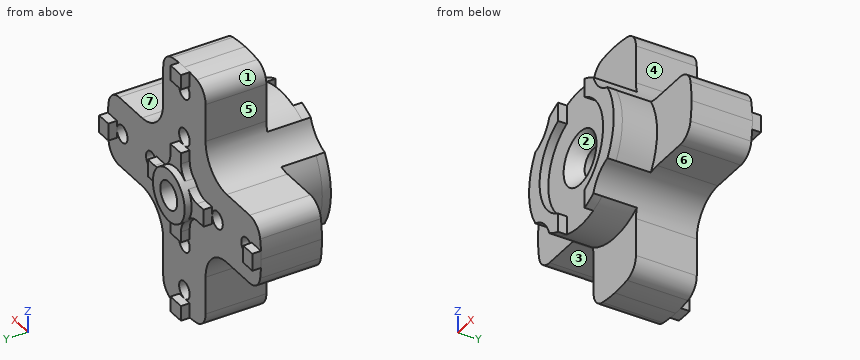
```python
from build123d import *

# Parameters (mm, degrees)
BOSS_EXTRUDE1_DEPTH   = 3.5
BOSS_EXTRUDE2_DEPTH   = 0.5
SKETCH6_R             = 4
BOSS_EXTRUDE4_DEPTH   = 2
FILLET1_R             = 1
SKETCH13_R            = 1.5
BOSS_EXTRUDE7_DEPTH   = 0.9
M2X0_4_TAPPED_HOLE1_D = 1.6
BOSS_EXTRUDE5_DEPTH   = 0.5
CUT_EXTRUDE1_START    = -3
SKETCH5_R             = 0.5
CUT_EXTRUDE1_DEPTH    = 3
SKETCH10_W            = 1
SKETCH10_H            = 3.75
SKETCH10_W_2          = 3.75
SKETCH10_H_2          = 1
CUT_EXTRUDE2_DEPTH    = 0.5
CHAMFER1_SIZE         = 0.75
FILLET2_R             = 2
CUT_EXTRUDE3_REACH    = 13.157
FILLET3_R             = 1


with BuildPart() as part:
    # Sketch3 → Boss-Extrude1 (new body)
    with BuildSketch(Plane(origin=(0, 0, 0), x_dir=(1, 0, 0), z_dir=(0, 1, 0))):
        with BuildLine():
            Line((-2, -6.968679932), (-2, -2))
            Line((-2, -2), (-6.968679932, -2))
            ThreePointArc((-6.968679932, -2), (-7.179325508, -1.009844169), (-7.25, 0))
            ThreePointArc((-7.25, 0), (-7.179325508, 1.009844169), (-6.968679932, 2))
            Line((-6.968679932, 2), (-2, 2))
            Line((-2, 2), (-2, 6.968679932))
            ThreePointArc((-2, 6.968679932), (-1.009844169, 7.179325508), (0, 7.25))
            ThreePointArc((0, 7.25), (1.009844169, 7.179325508), (2, 6.968679932))
            Line((2, 6.968679932), (2, 2))
            Line((2, 2), (6.968679932, 2))
            ThreePointArc((6.968679932, 2), (7.179325508, 1.009844169), (7.25, 0))
            ThreePointArc((7.25, 0), (7.179325508, -1.009844169), (6.968679932, -2))
            Line((6.968679932, -2), (2, -2))
            Line((2, -2), (2, -6.968679932))
            ThreePointArc((2, -6.968679932), (1.009844169, -7.179325508), (0, -7.25))
            ThreePointArc((0, -7.25), (-1.009844169, -7.179325508), (-2, -6.968679932))
        make_face()
    extrude(amount=BOSS_EXTRUDE1_DEPTH)

    # Sketch4 → Boss-Extrude2 (add)
    with BuildSketch(Plane(origin=(0, 3.5, 0), x_dir=(-1, 0, 0), z_dir=(0, 1, 0))):
        with BuildLine():
            Line((-0.5, 5.875), (-0.5, 7.232738071))
            ThreePointArc((-0.5, 7.232738071), (0, 7.25), (0.5, 7.232738071))
            Line((0.5, 7.232738071), (0.5, 5.875))
            ThreePointArc((0.5, 5.875), (0, 5.375), (-0.5, 5.875))
        make_face()
        with BuildLine():
            Line((0.5, 3.125), (0.5, 0.5))
            Line((0.5, 0.5), (3.125, 0.5))
            ThreePointArc((3.125, 0.5), (3.625, 0), (3.125, -0.5))
            Line((3.125, -0.5), (0.5, -0.5))
            Line((0.5, -0.5), (0.5, -3.125))
            ThreePointArc((0.5, -3.125), (0, -3.625), (-0.5, -3.125))
            Line((-0.5, -3.125), (-0.5, -0.5))
            Line((-0.5, -0.5), (-3.125, -0.5))
            ThreePointArc((-3.125, -0.5), (-3.625, 0), (-3.125, 0.5))
            Line((-3.125, 0.5), (-0.5, 0.5))
            Line((-0.5, 0.5), (-0.5, 3.125))
            ThreePointArc((-0.5, 3.125), (0, 3.625), (0.5, 3.125))
        make_face()
        with BuildLine():
            Line((5.875, 0.5), (7.232738071, 0.5))
            ThreePointArc((7.232738071, 0.5), (7.25, 0), (7.232738071, -0.5))
            Line((7.232738071, -0.5), (5.875, -0.5))
            ThreePointArc((5.875, -0.5), (5.375, 0), (5.875, 0.5))
        make_face()
        with BuildLine():
            Line((0.5, -5.875), (0.5, -7.232738071))
            ThreePointArc((0.5, -7.232738071), (0, -7.25), (-0.5, -7.232738071))
            Line((-0.5, -7.232738071), (-0.5, -5.875))
            ThreePointArc((-0.5, -5.875), (0, -5.375), (0.5, -5.875))
        make_face()
        with BuildLine():
            Line((-5.875, -0.5), (-7.232738071, -0.5))
            ThreePointArc((-7.232738071, -0.5), (-7.25, 0), (-7.232738071, 0.5))
            Line((-7.232738071, 0.5), (-5.875, 0.5))
            ThreePointArc((-5.875, 0.5), (-5.375, 0), (-5.875, -0.5))
        make_face()
    extrude(amount=BOSS_EXTRUDE2_DEPTH)

    # Sketch6 → Boss-Extrude4 (add)
    with BuildSketch(Plane.XZ):
        with Locations(Location((0, 0, 0), (0, 0, 120))):
            Circle(SKETCH6_R)
    extrude(amount=BOSS_EXTRUDE4_DEPTH)

    # Fillet1
    fillet1_edges = [part.edges().sort_by_distance(p)[0] for p in [
        (-2, 1.75, 6.968679932),
        (-6.968679932, 1.75, 2),
        (-6.968679932, 1.75, -2),
        (-2, 1.75, -6.968679932),
        (2, 1.75, -6.968679932),
        (6.968679932, 1.75, -2),
        (6.968679932, 1.75, 2),
        (2, 1.75, 6.968679932),
    ]]
    fillet(fillet1_edges, radius=FILLET1_R)

    # Sketch13 → Boss-Extrude7 (add)
    with BuildSketch(Plane(origin=(0, 3.5, 0), x_dir=(1, 0, 0), z_dir=(0, 1, 0))):
        with Locations(Location((0, 0, 0), (0, 0, 109.471220634))):
            Circle(SKETCH13_R)
    extrude(amount=BOSS_EXTRUDE7_DEPTH)

    # M2x0.4 Tapped Hole1 (through all)
    with Locations(Plane(origin=(0, -2, 0), x_dir=(-1, 0, 0), z_dir=(0, -1, 0))):
        with Locations((0, 0)):
            Hole(M2X0_4_TAPPED_HOLE1_D / 2)

    # Sketch9 → Boss-Extrude5 (add)
    with BuildSketch(Plane.XZ.offset(2)):
        with BuildLine():
            Line((-1.25, -2.727178029), (-1.25, -3.799671038))
            ThreePointArc((-1.25, -3.799671038), (-4, 0), (-1.25, 3.799671038))
            Line((-1.25, 3.799671038), (-1.25, 2.727178029))
            ThreePointArc((-1.25, 2.727178029), (-3, 0), (-1.25, -2.727178029))
        make_face()
        with BuildLine():
            Line((1.25, 2.727178029), (1.25, 3.799671038))
            ThreePointArc((1.25, 3.799671038), (4, 0), (1.25, -3.799671038))
            Line((1.25, -3.799671038), (1.25, -2.727178029))
            ThreePointArc((1.25, -2.727178029), (3, 0), (1.25, 2.727178029))
        make_face()
    extrude(amount=BOSS_EXTRUDE5_DEPTH)

    # Sketch5 → Cut-Extrude1 (cut)
    with BuildSketch(Plane(origin=(0, 4, 0), x_dir=(-1, 0, 0), z_dir=(0, 1, 0)).offset(CUT_EXTRUDE1_START)):
        with Locations(Location((0, 5.875, 0), (0, 0, 90))):
            Circle(SKETCH5_R)
        with Locations(Location((0, 3.125, 0), (0, 0, 90))):
            Circle(SKETCH5_R)
        with Locations(Location((5.875, 0, 0), (0, 0, 90))):
            Circle(SKETCH5_R)
        with Locations(Location((3.125, 0, 0), (0, 0, 90))):
            Circle(SKETCH5_R)
        with Locations(Location((0, -5.875, 0), (0, 0, 90))):
            Circle(SKETCH5_R)
        with Locations(Location((0, -3.125, 0), (0, 0, 90))):
            Circle(SKETCH5_R)
        with Locations(Location((-5.875, 0, 0), (0, 0, 90))):
            Circle(SKETCH5_R)
        with Locations(Location((-3.125, 0, 0), (0, 0, 90))):
            Circle(SKETCH5_R)
    extrude(amount=CUT_EXTRUDE1_DEPTH, mode=Mode.SUBTRACT)

    # Sketch10 → Cut-Extrude2 (cut)
    with BuildSketch(Plane(origin=(0, 4, 0), x_dir=(1, 0, 0), z_dir=(0, 1, 0))):
        with Locations((0, -4.5)):
            Rectangle(SKETCH10_W, SKETCH10_H)
        with Locations((-4.5, 0)):
            Rectangle(SKETCH10_W_2, SKETCH10_H_2)
        with Locations((0, 4.5)):
            Rectangle(SKETCH10_W, SKETCH10_H)
        with Locations((4.5, 0)):
            Rectangle(SKETCH10_W_2, SKETCH10_H_2)
    extrude(amount=-CUT_EXTRUDE2_DEPTH, mode=Mode.SUBTRACT)

    # Chamfer1
    chamfer1_edges = [part.edges().sort_by_distance(p)[0] for p in [
        (-0.8, -2, 0),
    ]]
    chamfer(chamfer1_edges, length=CHAMFER1_SIZE)

    # Fillet2
    # the kernel refuses this fillet: 2 mm, written as the material it adds along each edge
    with BuildSketch(Plane(origin=(-2, 0, 2), x_dir=(0, 0, 1), z_dir=(0, 1, 0)), Plane(origin=(-2, 0, -2), x_dir=(-1, 0, 0), z_dir=(0, 1, 0)), Plane(origin=(2, 0, -2), x_dir=(0, 0, -1), z_dir=(0, 1, 0)), Plane(origin=(2, 0, 2), x_dir=(1, 0, 0), z_dir=(0, 1, 0))) as fillet2_piece_1:
        with BuildLine():
            CenterArc((FILLET2_R, -FILLET2_R), FILLET2_R, 90, 90)
            Line((0, -FILLET2_R), (0, 0))
            Line((0, 0), (FILLET2_R, 0))
        make_face()
    extrude(amount=3.5)

    # Sketch11 → Cut-Extrude3 (cut, up to next)
    with BuildSketch(Plane(origin=(0, 0, 0), x_dir=(1, 0, 0), z_dir=(0, 1, 0)), mode=Mode.PRIVATE) as cut_extrude3_sk1:
        with BuildLine():
            ThreePointArc((3.411437828, -2.088562172), (2.585786438, -2.585786438), (2.088562172, -3.411437828))
            ThreePointArc((2.088562172, -3.411437828), (2.828427125, -2.828427125), (3.411437828, -2.088562172))
        make_face()
    cut_extrude3_tool1 = extrude(cut_extrude3_sk1.sketch, amount=-CUT_EXTRUDE3_REACH, mode=Mode.PRIVATE) & part.part
    # Sketch11 → Cut-Extrude3 (cut, up to next)
    with BuildSketch(Plane(origin=(0, 0, 0), x_dir=(1, 0, 0), z_dir=(0, 1, 0)), mode=Mode.PRIVATE) as cut_extrude3_sk2:
        with BuildLine():
            ThreePointArc((2.088562172, 3.411437828), (2.585786438, 2.585786438), (3.411437828, 2.088562172))
            ThreePointArc((3.411437828, 2.088562172), (2.828427125, 2.828427125), (2.088562172, 3.411437828))
        make_face()
    cut_extrude3_tool2 = extrude(cut_extrude3_sk2.sketch, amount=-CUT_EXTRUDE3_REACH, mode=Mode.PRIVATE) & part.part
    # Sketch11 → Cut-Extrude3 (cut, up to next)
    with BuildSketch(Plane(origin=(0, 0, 0), x_dir=(1, 0, 0), z_dir=(0, 1, 0)), mode=Mode.PRIVATE) as cut_extrude3_sk3:
        with BuildLine():
            ThreePointArc((-3.411437828, 2.088562172), (-2.585786438, 2.585786438), (-2.088562172, 3.411437828))
            ThreePointArc((-2.088562172, 3.411437828), (-2.828427125, 2.828427125), (-3.411437828, 2.088562172))
        make_face()
    cut_extrude3_tool3 = extrude(cut_extrude3_sk3.sketch, amount=-CUT_EXTRUDE3_REACH, mode=Mode.PRIVATE) & part.part
    # Sketch11 → Cut-Extrude3 (cut, up to next)
    with BuildSketch(Plane(origin=(0, 0, 0), x_dir=(1, 0, 0), z_dir=(0, 1, 0)), mode=Mode.PRIVATE) as cut_extrude3_sk4:
        with BuildLine():
            ThreePointArc((-2.088562172, -3.411437828), (-2.585786438, -2.585786438), (-3.411437828, -2.088562172))
            ThreePointArc((-3.411437828, -2.088562172), (-2.828427125, -2.828427125), (-2.088562172, -3.411437828))
        make_face()
    cut_extrude3_tool4 = extrude(cut_extrude3_sk4.sketch, amount=-CUT_EXTRUDE3_REACH, mode=Mode.PRIVATE) & part.part
    add(cut_extrude3_tool1.solids().sort_by_distance((2.71527, 0, 2.71527))[0], mode=Mode.SUBTRACT)
    add(cut_extrude3_tool2.solids().sort_by_distance((2.71527, 0, -2.71527))[0], mode=Mode.SUBTRACT)
    add(cut_extrude3_tool3.solids().sort_by_distance((-2.71527, 0, -2.71527))[0], mode=Mode.SUBTRACT)
    add(cut_extrude3_tool4.solids().sort_by_distance((-2.71527, 0, 2.71527))[0], mode=Mode.SUBTRACT)

    # Fillet3
    # the kernel refuses this fillet: 1 mm, written as the material it adds along each edge
    with BuildSketch(Plane(origin=(-1.414213562, 4, -0.5), x_dir=(0.4720978535930623, 0, -0.8815461511644318), z_dir=(0, -1, 0)), Plane(origin=(-0.5, 4, 1.414213562), x_dir=(-0.8815461511644338, 0, -0.47209785359305884), z_dir=(0, -1, 0)), Plane(origin=(1.414213562, 4, 0.5), x_dir=(-0.47209785359305845, 0, 0.881546151164434), z_dir=(0, -1, 0)), Plane(origin=(0.5, 4, -1.414213562), x_dir=(0.8815461511644322, 0, 0.4720978535930617), z_dir=(0, -1, 0)), Plane(origin=(-0.5, 2.035533906, -1.414213562), x_dir=(-0.8815461511644342, 0, 0.47209785359305795), z_dir=(0, 1, 0))) as fillet3_piece_1:
        with BuildLine():
            CenterArc((0.604997631, -0.988495633), FILLET3_R, 98.699338506, 53.130102354)
            Line((-0.27654852, -0.516397779), (0, 0))
            ThreePointArc((0, 0), (0.226874112, -0.01725655), (0.453748223, 0))
        make_face()
    extrude(amount=1.964466094)
    with BuildSketch(Plane(origin=(-1.414213562, 4, 0.5), x_dir=(0.472097853593057, 0, 0.8815461511644348), z_dir=(0, -1, 0)), Plane(origin=(0.5, 4, 1.414213562), x_dir=(0.8815461511644329, 0, -0.47209785359306067), z_dir=(0, -1, 0))) as fillet3_piece_2:
        with BuildLine():
            CenterArc((0.604997631, 0.988495633), FILLET3_R, 208.17055914, 53.130102354)
            Line((-0.27654852, 0.516397779), (0, 0))
            ThreePointArc((0, 0), (0.226874112, 0.01725655), (0.453748223, 0))
        make_face()
    extrude(amount=1.964466094)
    with BuildSketch(Plane(origin=(1.414213562, 4, -0.5), x_dir=(1, 0, 0), z_dir=(0, -1, 0))) as fillet3_piece_3:
        with BuildLine():
            CenterArc((0.585786438, -1), FILLET3_R, 90, 53.130102354)
            ThreePointArc((-0.214213562, -0.4), (-0.091894336, -0.20814678), (0, 0))
            Line((0, 0), (0.585786438, 0))
        make_face()
    extrude(amount=1.964466094)


solid = part.part
```
Model file for the job. Use its own axes, mm. Face numbers are marked on the shaded views. A direction names the side the tool comes from. Give positions to 0.01 mm unless a question says otherwise; leave off trailing zeros. Loops run counter-clockwise (first coordinate to the right, second up) from the corner with the lowest first, then second, coordinate; pieces in that order, holes last. Notation, with made-up numbers: (19.25, 32.25) - (46.25, 32.25) arc R20 cw to (46.25, 70.25) - close; hole circle Ø4 at (68, -28). An arc over 180 degrees is marked (long way). One line per item, written item: value. Start each with the question number.
1. Probe L1, parallel to Y at x = -5.75, z = -0.25; L2, parallel to Y at x = 1.5, z = -3.25; L3, parallel to Z at x = -5.25, y = 2.25. List the from-to ranges inside material, lowest first. Write a range as from..to.
2. Pull direction Z, two halves, no side cores. Call the marked faces 1, 2, 3 and 4: pulls with the +Z half, pulls with the -Z half, needs draft (parallel to the pull), parting line crosses it, or undercut.
3. Which spindle directions (+Z, -Z, +X, -X, +Y, -Y) get a long thin tool onto all of the face, cutting with end or side? Do the marked faces 5, 6 and 7. Say none if no direction does.
4. Slice it at C-C (y = 3). Give the number of separate pieces and of enclosed holes in the cut face, plus the area to 3 significant figures.
5. Slice it at B-B (y = 0.5). List the corners of the cut face in (x, z).
6. Slice it at A-A (y = -0.5). List the corners of the cut face in (x, z), plus the area to 3 significant figures.
7. Pin check, flat tips, straight feed: pin 1 (2 mm diameter, centred on x = -1.5, z = 5, fed in from +Y); pin 2 (2 mm diameter, centred on x = -5, y = 2, fed in from -Z); pin 3 (1.1 mm diameter, centred on x = -3, z = 0, fed in from +Y). Stop position of each tip, or through.
Solution:
1. L1: y = 0..1
1. L2: y = -2.5..3.5
1. L3: z = -2..2
2. face 1: pulls with the +Z half
2. face 2: undercut
2. face 3: pulls with the -Z half
2. face 4: needs draft
3. face 5: +Z, -X, +Y, -Y
3. face 6: -Z, +X, +Y, -Y
3. face 7: +Z, +X, +Y, -Y
4. separate pieces: 1
4. enclosed holes: 9
4. area: 92.6 mm^2
5. outline: (-7.16, -1.16) arc R1 ccw to (-6.17, -2) - (-4, -2) arc R2 cw to (-2, -4) - (-2, -6.17) arc R1 ccw to (-1.16, -7.16) arc R7.25 ccw to (1.16, -7.16) arc R1 ccw to (2, -6.17) - (2, -4) arc R2 cw to (4, -2) - (6.17, -2) arc R1 ccw to (7.16, -1.16) arc R7.25 ccw to (7.16, 1.16) arc R1 ccw to (6.17, 2) - (4, 2) arc R2 cw to (2, 4) - (2, 6.17) arc R1 ccw to (1.16, 7.16) arc R7.25 ccw to (-1.16, 7.16) arc R1 ccw to (-2, 6.17) - (-2, 4) arc R2 cw to (-4, 2) - (-6.17, 2) arc R1 ccw to (-7.16, 1.16) arc R7.25 ccw to start; hole circle Ø1.6 at (0, 0)
6. outline: (-3.41, -2.09) arc R2 cw to (-2.09, -3.41) arc R4 ccw to (2.09, -3.41) arc R2 cw to (3.41, -2.09) arc R4 ccw to (3.41, 2.09) arc R2 cw to (2.09, 3.41) arc R4 ccw to (-2.09, 3.41) arc R2 cw to (-3.41, 2.09) arc R4 ccw to start; hole circle Ø1.6 at (0, 0)
6. area: 46.5 mm^2
7. pin 1: stops at y = 3.5
7. pin 2: stops at z = -2
7. pin 3: stops at y = 4
